Build history of the part. All positions in model axes, mm. Face numbers are marked on the shaded views. A direction names the side the tool comes from. Coordinates: 2 decimals unless noted, no trailing zeros. Order: outer loops, then holes, each group sorted by start corner. A loop starts at its lowest first (then second) coordinate and runs counter-clockwise, first axis right, second up. Notation, with made-up numbers: M 11,22 L 20,22 A23 ccw 20,32 Z; hole C -37,-25 d5. An arc over 180 degrees is marked long. Use a Markdown table: item, result. Add a question column.
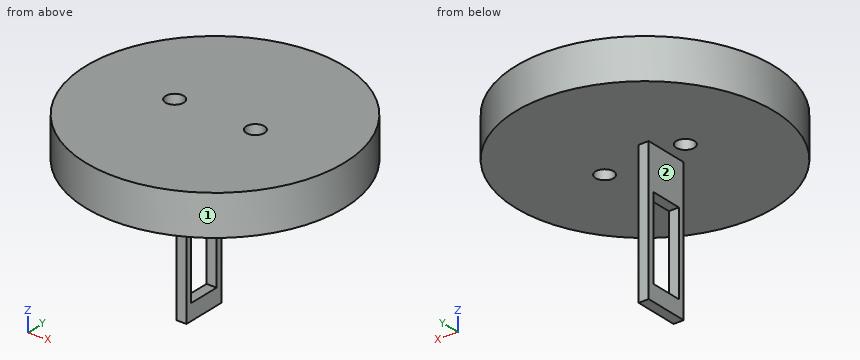
from build123d import *

# Parameters (mm, degrees)
SKETCH004_R     = 64.00438
PAD003_DEPTH    = 20
SKETCH006_R     = 4.5
POCKET001_DEPTH = 20
SKETCH005_R     = 4.5
POCKET002_DEPTH = 20
SKETCH007_W     = 5
SKETCH007_H     = 22
PAD004_DEPTH    = 70
SKETCH008_W     = 16
SKETCH008_H     = 40.7
POCKET003_DEPTH = 5


with BuildPart() as part:
    # Sketch004 → Pad003 (new body)
    with BuildSketch(Plane.XY):
        Circle(SKETCH004_R)
    extrude(amount=PAD003_DEPTH)

    # Sketch006 → Pocket001 (cut)
    with BuildSketch(Plane.XY):
        with Locations((20, 0)):
            Circle(SKETCH006_R)
    extrude(amount=POCKET001_DEPTH, mode=Mode.SUBTRACT)

    # Sketch005 → Pocket002 (cut)
    with BuildSketch(Plane.XY):
        with Locations((-20, 0)):
            Circle(SKETCH005_R)
    extrude(amount=POCKET002_DEPTH, mode=Mode.SUBTRACT)

    # Sketch007 → Pad004 (join)
    with BuildSketch(Plane.XY):
        with Locations((-8, 0)):
            Rectangle(SKETCH007_W, SKETCH007_H)
    extrude(amount=-PAD004_DEPTH)

    # Sketch008 (on Face7 of Pad004) → Pocket003 (cut)
    with BuildSketch(Plane.YZ.offset(-5.5)):
        with Locations((0, -41.65)):
            Rectangle(SKETCH008_W, SKETCH008_H)
    extrude(amount=-POCKET003_DEPTH, mode=Mode.SUBTRACT)


with BuildPart() as part_1:
    # Body001 placement: moved
    add(part.part.moved(Location((-57, 6, -43))))


solid = part_1.part
(1) Drop flat-ended pins along their axis: P1, Ø4, axis at x = -66, z = -63, coming from the -Y side; P2, Ø3, axis at x = -95.5, y = -31, coming from the -Z side; P3, Ø17.5, axis at y = 4, z = -89.5, coming from the +X side. Give the stop position or say it passes through.
(2) Drill centre lines: line 1 along Z through (x, y) = (-90, -37); line 2 along Y through (x, z) = (-77, -33.25); line 3 along Y through (x, z) = (-36, -34). Where is each one in solid material? Low to high. Write a range as from..to.
(3) Which spindle directions (+Z, -Z, +X, -X, +Y, -Y) get a long thin tool onto all of the face, cutting with end or side? Do the marked faces 1 and 2. Say none if no direction does.
(4) Slice it at B-B on x = -77. Give the cut face in (y, z).
(5) Slice it at A-A on z = -76. Give the cut face in (x, y).
(6) Slice it at D-D on x = -57. Give the cut face in (y, z), and give its area (3 significant figures).
(7) Slice it at C-C on y = 6. Give the cut face in (x, z).
Solutions:
| question | item | result |
|---|---|---|
| 1 | P1 | y = -5 |
| 1 | P2 | z = -43 |
| 1 | P3 | x = -62.5 |
| 2 | line 1 | -43..-23 |
| 2 | line 2 | -54.8..1.5, 10.5..66.8 |
| 2 | line 3 | -54.46..1.61, 10.39..66.46 |
| 3 | face 1 | +Z, -Z |
| 3 | face 2 | -Z, -X, +Y, -Y |
| 4 | outline | M -54.8,-43 L 1.5,-43 L 1.5,-23 L -54.8,-23 Z; M 10.5,-43 L 66.8,-43 L 66.8,-23 L 10.5,-23 Z |
| 5 | outline | M -67.5,-5 L -62.5,-5 L -62.5,-2 L -67.5,-2 Z; M -67.5,14 L -62.5,14 L -62.5,17 L -67.5,17 Z |
| 6 | outline | M -58,-43 L 70,-43 L 70,-23 L -58,-23 Z |
| 6 | area | 2,560 mm² |
| 7 | outline | M -121,-43 L -81.5,-43 L -81.5,-23 L -121,-23 Z; M -72.5,-43 L -67.5,-43 L -67.5,-64.3 L -62.5,-64.3 L -62.5,-43 L -41.5,-43 L -41.5,-23 L -72.5,-23 Z; M -67.5,-113 L -62.5,-113 L -62.5,-105 L -67.5,-105 Z; M -32.5,-43 L 7,-43 L 7,-23 L -32.5,-23 Z |
